Job drawing, mm, ordinate dimensions from the low corner. One solid piece. A direction names the side the tool comes from. Give positions to 0.01 mm unless a question says otherwise; leave off trailing zeros. Loops run counter-clockwise (first coordinate to the right, second up) from the corner with the lowest first, then second, coordinate; pieces in that order, holes last.
Item 1: Saw through at D-D on x = 12.5. Give the cut face in (y, z).
Item 2: Saw through at C-C on x = 75. Give the cut face in (y, z), plus the area to 3 significant figures.
Item 3: Drop flat-ended pins along their axis: P1, Ø1, axis at x = 15, z = 36, coming from the +Y side; P2, Ø5, axis at y = 93, z = 32, coming from the +X side; P3, Ø4, axis at x = 16.5, z = 64.5, coming from the -Y side. Give the stop position or say it passes through.
Item 4: Saw through at B-B on y = 61.5. Give the cut face in (x, z) (1 decimal), plus the area to 3 significant figures.
Item 5: Probe probe 1 along Y at (x, z) = (46, 21) (1 decimal); probe 2 along Y at (x, z) = (54, 59); probe 3 along X at (y, z) = (73.5, 9) (1 decimal). List the from-to ranges inside material, lowest first.
Item 6: Saw through at A-A on z = 44. Give the number of separate pieces and of enclosed holes in the cut face, plus the area to 3 significant figures.
Item 7: Which spindle directions (+Z, -Z, +X, -X, +Y, -Y) get a long thin tool onto all of the face, cutting with end or side? Do the marked faces 1 and 2. Say none if no direction does.
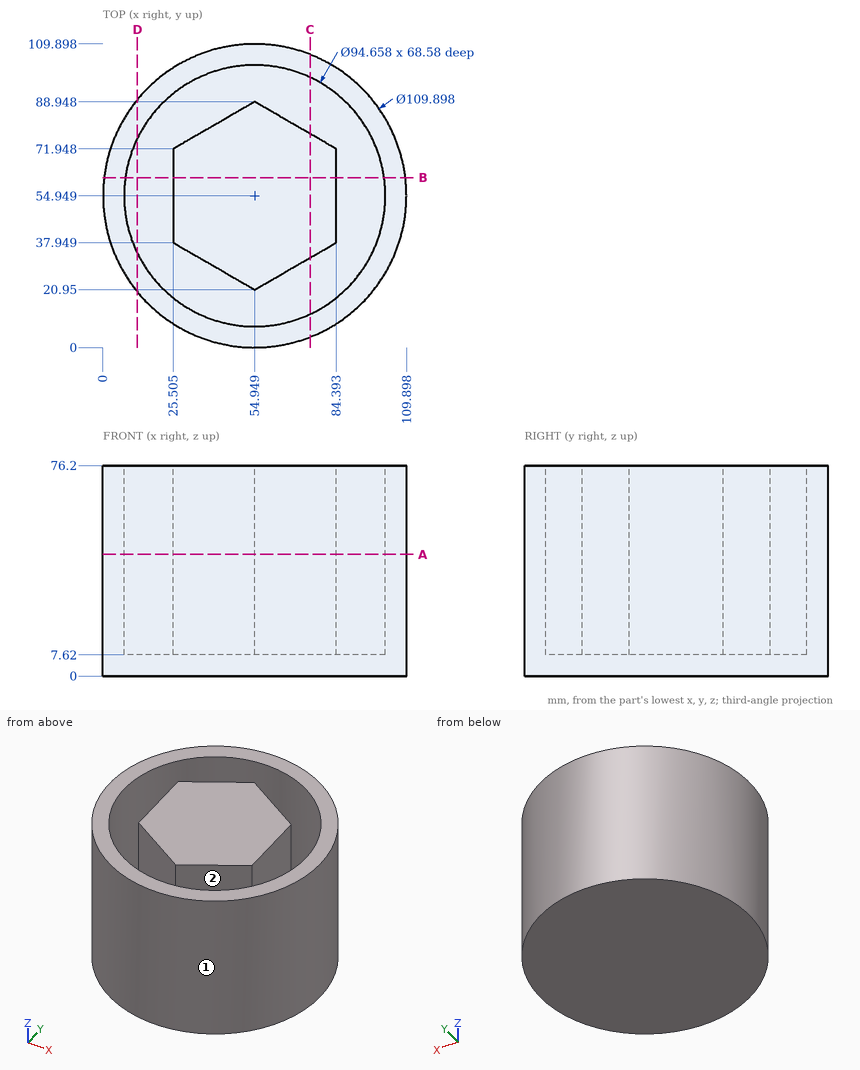
Results below:
1. outline: (20.06, 0) - (89.84, 0) - (89.84, 76.2) - (75.88, 76.2) - (75.88, 7.62) - (34.02, 7.62) - (34.02, 76.2) - (20.06, 76.2) - close
2. outline: (3.79, 0) - (106.11, 0) - (106.11, 76.2) - (97.82, 76.2) - (97.82, 7.62) - (77.37, 7.62) - (77.37, 76.2) - (32.53, 76.2) - (32.53, 7.62) - (12.08, 7.62) - (12.08, 76.2) - (3.79, 76.2) - close
2. area: 4,990 mm2
3. P1: stops at y = 93.2
3. P2: stops at x = 96.85
3. P3: stops at y = 13.83
4. outline: (0.4, 0) - (109.5, 0) - (109.5, 76.2) - (101.8, 76.2) - (101.8, 7.6) - (84.4, 7.6) - (84.4, 76.2) - (25.5, 76.2) - (25.5, 7.6) - (8.1, 7.6) - (8.1, 76.2) - (0.4, 76.2) - close
4. area: 5,920 mm2
5. probe 1: y = 0.7 to 8.5, 26.1 to 83.8, 101.4 to 109.2
5. probe 2: y = 0.01 to 7.63, 21.5 to 88.4, 102.27 to 109.89
5. probe 3: x = 3.2 to 11.4, 28.2 to 81.7, 98.5 to 106.7
6. separate pieces: 2
6. enclosed holes: 1
6. area: 5,450 mm2
7. face 1: +Z, -Z
7. face 2: +Z
